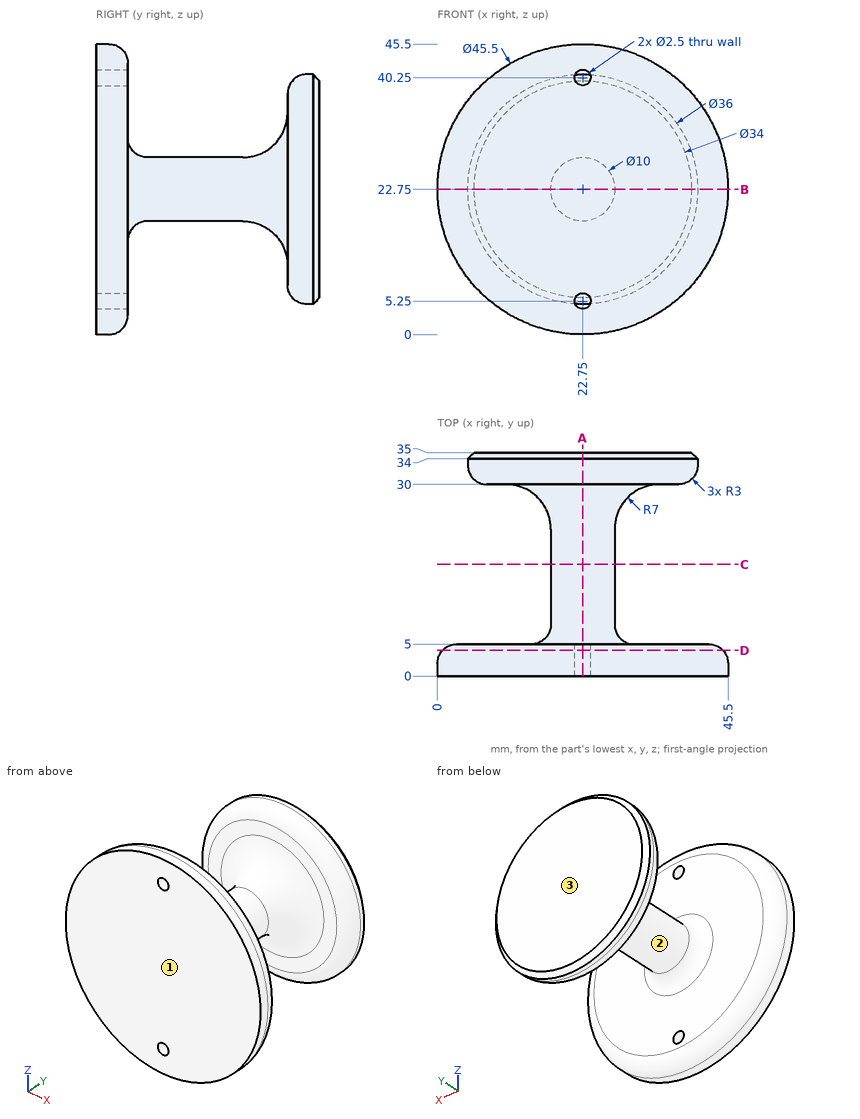
Here's the drawing with two shaded views (mm, measured from the low corner). I have some questions. Give positions to 0.01 mm unless a question says otherwise; leave off trailing zeros. Loops run counter-clockwise (first coordinate to the right, second up) from the corner with the lowest first, then second, coordinate; pieces in that order, holes last. Notation, with made-up numbers: M -35,16 L 7,16 A27 cw 7,36 Z; hole C 82,62 d4. An arc over 180 degrees is marked long. One line per item, written item: value. Start each with the question number.
1) I'm going to push flat-ended pins straight in: pin 1 (5 mm diameter, centred on x = 26.5, y = 13.5, fed in from -Z); pin 2 (12 mm diameter, centred on y = 4.5, z = 26, fed in from +X); pin 3 (4 mm diameter, centred on y = 15, z = 17, fed in from -X); pin 4 (8 mm diameter, centred on y = 7, z = 33.5, fed in from -X). Where does each tip first touch, or does it pass through?
2) If we section it at D-D, the plane y = 4: Write out the boundary of the cut face in (x, z).
3) If we section it at A-A, the plane x = 22.75: Give the number of separate pieces and of enclosed holes in the cut face, and give its area (3 significant figures).
4) If I drill on line 1 (Y direction, x = 10.5, z = 22); line 2 (Z direction, x = 22, y = 1); line 3 (Y direction, x = 24.5, z = 6.5), over which ranges is the centre line in solid material (lowest first)? Write a range as [from, to].
5) If we section it at C-C, the plane y = 17.5: Write out the boundary of the cut face in (x, z), and give its area (3 significant figures).
6) Thinking about a two-plate mould opening in Y: for the marked faces 1, 2 and 3, which applies, +Y half, -Y half, draft (parallel to the pull), parting line (faces both ways), or undercut?
7) If we section it at B-B, the plane z = 22.75: Write out the boundary of the cut face in (x, y), and give its area (3 significant figures).
Completed:
1. pin 1: stops at z = 17.91
1. pin 2: stops at x = 45.5
1. pin 3: stops at x = 19.44
1. pin 4: stops at x = 2.21
2. outline: C 22.75,22.75 d43.97; hole C 22.75,5.25 d2.5; hole C 22.75,40.25 d2.5
3. separate pieces: 3
3. enclosed holes: 0
3. area: 649 mm^2
4. line 1: y = [0, 5], [30, 35]
4. line 2: z = [0.01, 4.25], [6.25, 39.25], [41.25, 45.49]
4. line 3: y = [0, 5], [30.32, 35]
5. outline: C 22.75,22.75 d10
5. area: 78.5 mm^2
6. face 1: -Y half
6. face 2: undercut
6. face 3: +Y half
7. outline: M 0,0 L 45.5,0 L 45.5,2 A3 ccw 42.5,5 L 30.75,5 A3 cw 27.75,8 L 27.75,23 A7 cw 34.75,30 L 37.75,30 A3 ccw 40.75,33 L 40.75,34 L 39.75,35 L 5.75,35 L 4.75,34 L 4.75,33 A3 ccw 7.75,30 L 10.75,30 A7 cw 17.75,23 L 17.75,8 A3 cw 14.75,5 L 3,5 A3 ccw 0,2 Z
7. area: 674 mm^2
